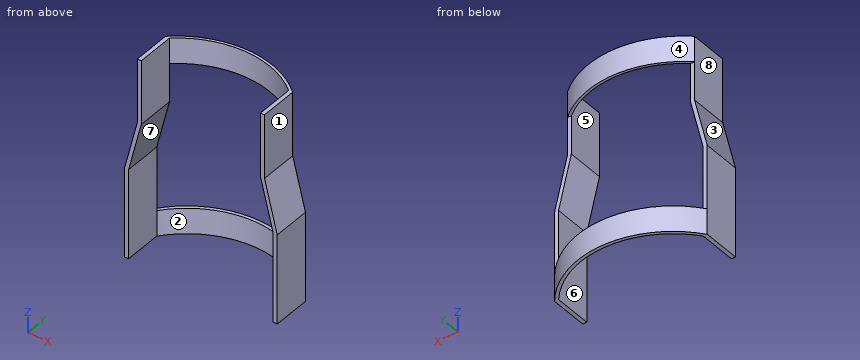
```python
from build123d import *

# Parameters (mm, degrees)
F1_DEPTH = 25.4
F2_DEPTH = 38.1
F4_DEPTH = 38.1
F7_DEPTH = 25.4


# Not quite as in the source:
# - a pattern or mirror of a feature is missing from the dataset's text; its kind, count and spacing are read off the source's solid


with BuildPart() as f1:
    # F0 (on Top) → F1 (new body)
    with BuildSketch(Plane.XY):
        with BuildLine():
            Line((148.3919879557, 0), (152.4, 0))
            ThreePointArc((152.4, 0), (76.2, 38.1), (0, 0))
            Line((0, 0), (4.0080120443, 0))
            ThreePointArc((4.0080120443, 0), (76.2, 34.925), (148.3919879557, 0))
        make_face()
    extrude(amount=F1_DEPTH)

    # F2 (add): faces of the model
    f2_faces = [f1.faces().sort_by_distance(p)[0] for p in [
        (150.3959939779, 0, 12.7),
        (2.0040060221, 0, 12.7),
    ]]
    extrude(f2_faces, amount=F2_DEPTH)

    # F3 (on Front) → F4 (join)
    with BuildSketch(Plane.XZ):
        Polygon((0, 25.4), (4.0080120443, 25.4), (4.0080120443, 88.9), (16.7080120443, 139.7), (16.7080120443, 203.2), (12.7, 203.2), (12.7, 139.7), (0, 88.9), align=None)
    f4 = extrude(amount=F4_DEPTH)

    # F4_copies: F4 across plane
    add(f4.mirror(Plane(origin=(76.2, 0, 0), x_dir=(0, 0, 1), z_dir=(1, 0, 0))))

    # F6 (on face) → F7 (join)
    with BuildSketch(Plane.XY.offset(203.2)):
        with BuildLine():
            ThreePointArc((16.7080120443, 0), (76.2, 21.631021226), (135.6919879557, 0))
            Line((135.6919879557, 0), (139.7, 0))
            ThreePointArc((139.7, 0), (76.2, 24.2548417144), (12.7, 0))
            Line((12.7, 0), (16.7080120443, 0))
        make_face()
    extrude(amount=-F7_DEPTH)


solid = f1.part
```
Read the model definition and answer for the solid it produces. Units are mm, in the model's axes. Face numbers are marked on the shaded views. A direction names the side the tool comes from. Give positions to 0.01 mm unless a question says otherwise; leave off trailing zeros. Loops run counter-clockwise (first coordinate to the right, second up) from the corner with the lowest first, then second, coordinate; pieces in that order, holes last.
Item 1: For the marked faces 5, 6, 7 and 8, determine the directions among +Z, -Z, +X, -X, +Y, -Y from which every point of the face is accessible in a straight line to the end or side of a thin tool.
Item 2: The part is cut by section B-B (x = 132.5). Write down the section's boundary in (y, z) (3 decimals).
Item 3: The mould has two halves that part along X. Classify the marked faces 1, 2, 3 and 4: released by +X, released by -X, zero draft, split by the parting line, or undercut.
Item 4: Find the intervals of material crossed by line 1 along X through (y, z) = (-35, 30); line 2 along X through (y, z) = (-31.5, 194); line 3 along Y through (x, z) = (136, 155.5), in increasing order.
Item 5: The part is cut by section D-D (y = 12.5). Write down the section's boundary in (x, z), and give its area (3 significant figures).
Item 6: The part is cut by section A-A (y = -17.5). Write down the section's boundary in (x, z).
Item 7: Each of these flat-tipped pins is pushed along its axis until it touches: pin 1 Ø18.5 at (x, z) = (142.5, 101) entering from +Y; pin 2 Ø10 at (x, y) = (56, 19.5) entering from -Z; pin 3 Ø10 at (x, z) = (116.5, 28.5) entering from -Y. Where does it stop, or does it pass through?
Item 8: The part is cut by section C-C (z = 119). Write down the section's boundary in (x, y) (3 decimals), and give its area (3 significant figures).
Taken from the geometry:
1. face 5: +Z, -Z, -Y
1. face 6: -Z, -Y
1. face 7: -Z, +Y, -Y
1. face 8: +Z, -X, +Y, -Y
2. outline: (2.557, 177.8) - (5.835, 177.8) - (5.835, 203.2) - (2.557, 203.2) - close; (15.707, 0) - (19.68, 0) - (19.68, 25.4) - (15.707, 25.4) - close
3. face 1: released by +X
3. face 2: undercut
3. face 3: released by -X
3. face 4: split by the parting line
4. line 1: x = 0 to 4.01, 148.39 to 152.4
4. line 2: x = 12.7 to 16.71, 135.69 to 139.7
4. line 3: y = -38.1 to 0
5. outline: (11.23, 0) - (15.98, 0) - (15.98, 25.4) - (11.23, 25.4) - close; (30.36, 177.8) - (36.1, 177.8) - (36.1, 203.2) - (30.36, 203.2) - close; (116.3, 177.8) - (122.04, 177.8) - (122.04, 203.2) - (116.3, 203.2) - close; (136.42, 0) - (141.17, 0) - (141.17, 25.4) - (136.42, 25.4) - close
5. area: 533 mm2
6. outline: (0, 0) - (4.01, 0) - (4.01, 88.9) - (16.71, 139.7) - (16.71, 203.2) - (12.7, 203.2) - (12.7, 139.7) - (0, 88.9) - close; (135.69, 139.7) - (148.39, 88.9) - (148.39, 0) - (152.4, 0) - (152.4, 88.9) - (139.7, 139.7) - (139.7, 203.2) - (135.69, 203.2) - close
7. pin 1: stops at y = 0
7. pin 2: stops at z = 177.8
7. pin 3: stops at y = 23.61
8. outline: (7.525, -38.1) - (11.533, -38.1) - (11.533, 0) - (7.525, 0) - close; (140.867, -38.1) - (144.875, -38.1) - (144.875, 0) - (140.867, 0) - close
8. area: 305 mm2
